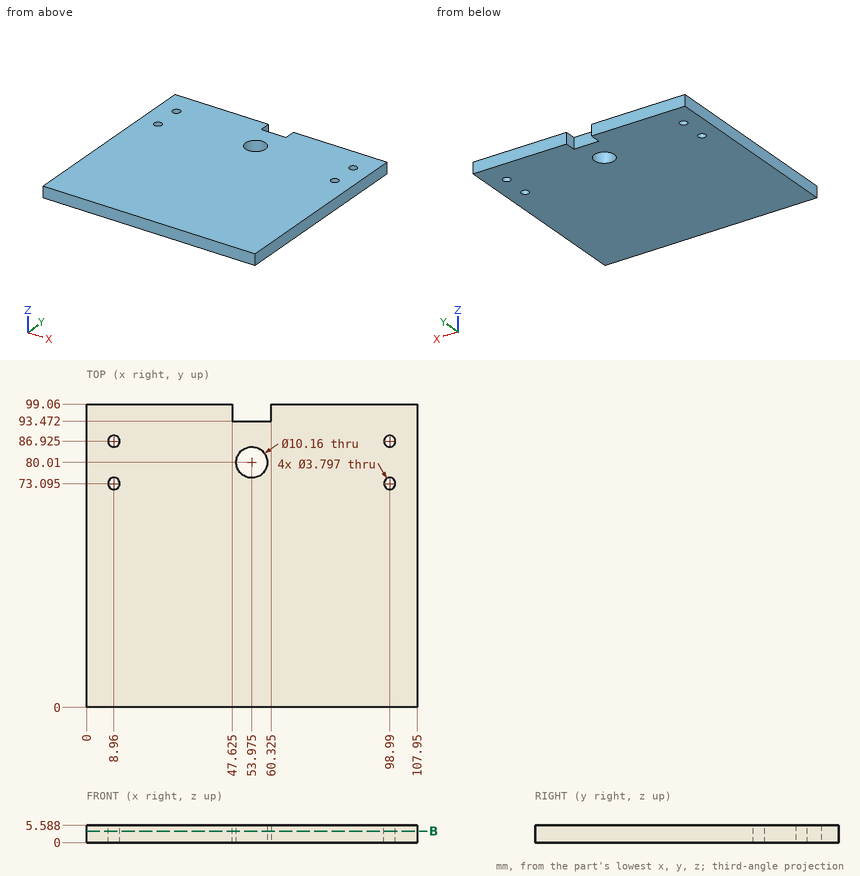
Design review of the part shown in the three views and the two pictorial views. Dimensions are in mm from the part's minimum x, y and z. Give positions to 0.01 mm unless a question says otherwise; leave off trailing zeros.
Item 1: Wall thickness on probe 1 along Y at (x, z) = (54, 4.05); probe 2 along Y at (x, z) = (7.5, 2.75); probe 3 along X at (y, z) = (77.5, 1.1): over which ranges is each line inside the solid? List them lowest first.
Item 2: Insertion check: P1, Ø6, axis at x = 98.99, y = 86.92, coming from the -Z side. The pin has a flat end and moves straight along its axis. Give the tip position at first contact, or say it passes through.
Item 3: Take a section at B-B (z = 3.75). Give the number of separate pieces and of enclosed holes in the cut face, and give its area (3 significant figures).
Established:
1. probe 1: y = 0 to 74.93, 85.09 to 93.47
1. probe 2: y = 0 to 71.88, 74.31 to 85.71, 88.14 to 99.06
1. probe 3: x = 0 to 49.56, 58.39 to 107.95
2. P1: stops at z = 0
3. separate pieces: 1
3. enclosed holes: 5
3. area: 10,500 mm2
